Autodesk Inventor part; units mm, degrees
ref_plane "YZ Plane" through (0, 0, 0) normal (1, 0, 0) x (0, 1, 0)
ref_plane "XZ Plane" through (0, 0, 0) normal (0, 1, 0) x (-1, 0, 0)
ref_plane "XY Plane" through (0, 0, 0) normal (0, 0, 1) x (1, 0, 0)
sketch "スケッチ1" plane through (0, 0, 0) normal (0, 0, 1) x (1, 0, 0)
  line L0 (0, 0) -> (40, 0)
  line L1 (40, 0) -> (40, 318)
  line L2 (40, 318) -> (0, 318)
  line L3 (0, 318) -> (0, 0)
  line L4 (0, 218) -> (112.7627, 152.8964)
  line L5 (112.7627, 152.8964) -> (132.7627, 187.5375)
  line L6 (132.7627, 187.5375) -> (40, 241.094)
  point P0 (40, 218)
  point P1 (40, 194.906)
  point P2 (20, 318)
  point P3 (122.7627, 170.2169)
  point P4 (20, 258)
  dimension "d0" = 40
  dimension "d1" = 318
  dimension "d69" = 40
  dimension "d70" = 60
  dimension "d91" = 20
  dimension "d92" = 100
  dimension "d93" = 180
  dimension "d96" = 20
  dimension "d97" = 60
extrude "押し出し1" add sketch "スケッチ1" along normal blind 19.6 contours L3 L2 L1 L4 | L1 L6 L5 L4
sketch "スケッチ6" plane through (0, 0, 19.6) normal (0, 0, 1) x (1, 0, 0)
  circle A0 centre (20, 258) radius 4
  line L0 (40, 318) -> (0, 318)
  line L1 (40, 241.094) -> (40, 318)
  circle A1 centre (20, 20) radius 1.2295
  circle A2 centre (20, 10) radius 1.2295
  line L2 (0, 0) -> (40, 0)
  circle A3 centre (20, 298) radius 4
  point P0 (20, 318)
  point P1 (40, 190.8114)
  point P2 (30, 0)
  dimension "d42" = 8
  dimension "d44" = 20
  dimension "d45" = 2.459
  dimension "d46" = 2.459
  dimension "d47" = 10
  dimension "d48" = 10
  dimension "d49" = 20
  dimension "d50" = 20
  dimension "d53" = 8
  dimension "d54" = 20
  dimension "d55" = 40
  dimension "d56" = 20
extrude "押し出し4" cut sketch "スケッチ6" against normal through all
sketch "スケッチ8" plane through (0, 0, 0) normal (-1, 0, 0) x (0, 0, 1)
  line L0 (0, 318) -> (19.6, 318)
  line L1 (5, 318) -> (14.6, 318)
  line L2 (14.6, 318) -> (14.6, 278)
  line L3 (14.6, 278) -> (5, 278)
  line L4 (5, 278) -> (5, 318)
  line L5 (0, 318) -> (0, 0)
  dimension "d57" = 5
  dimension "d58" = 9.6
  dimension "d59" = 40
  dimension "d98" = 19.6
extrude "押し出し5" cut sketch "スケッチ8" against normal through all
fillet "フィレット1" radius 20 4 edges at (40, 318, 17.1) (40, 318, 2.5) (0, 318, 2.5) (0, 318, 17.1)
fillet "フィレット2" radius 40 2 edges at (0, 218, 9.8) (40, 241.094, 9.8)
sketch "スケッチ9" plane through (0, 0, 19.6) normal (0, 0, 1) x (1, 0, 0)
  line L0 (20, 206.453) -> (112.7627, 152.8964)
  line L1 (132.7627, 187.5375) -> (60, 229.547)
  line L2 (112.7627, 152.8964) -> (132.7627, 187.5375)
  line L3 (132.7627, 187.5375) -> (112.7627, 152.8964)
  line L4 (66.3813, 179.6747) -> (112.7627, 152.8964)
  line L5 (132.7627, 187.5375) -> (166.773, 167.9016)
  line L6 (115.1204, 126.9801) -> (133.5174, 158.8446)
  line L7 (141.7531, 173.1092) -> (128.7627, 180.6092)
  line L8 (112.7627, 152.8964) -> (20, 206.453)
  line L9 (132.7627, 187.5375) -> (60, 229.547)
  line L10 (115.1204, 126.9801) -> (125.7531, 145.3964)
  line L11 (133.5174, 158.8446) -> (145.7531, 180.0375)
  line L12 (116.7627, 159.8246) -> (129.7531, 152.3246)
  line L13 (66.3813, 179.6747) -> (129.7531, 152.3246)
  line L14 (66.3813, 179.6747) -> (86.3813, 214.3157)
  line L15 (86.3813, 214.3157) -> (141.7531, 173.1092)
  point P0 (0, 0)
  point P1 (254.4532, 80.329)
  point P2 (128.7627, 180.6092)
  point P3 (123.2579, 156.0746)
  point P4 (86.3813, 214.3157)
  point P5 (40, 194.906)
  point P6 (115.8875, 158.3088)
  point P7 (129.6379, 182.1251)
  dimension "d80" = 24
  dimension "d81" = 40
  dimension "d83" = 15
  dimension "d84" = 8
  dimension "d90" = 24
extrude "押し出し6" cut sketch "スケッチ9" against normal through all contours L13 L2 L0 | L1 L2 L15
sketch "スケッチ11" plane through (104.9897, 139.4332, 24) normal (0.8660254, -0.5, 0) x (0, 0, -1)
  line L0 (4.4, 21.7957) -> (4.4, 49.2964)
  line L1 (24, 21.7957) -> (24, 49.2964)
  line L2 (0, 24) -> (24, 24)
  line L3 (24, 24) -> (24, 0)
  line L4 (24, 0) -> (0, 0)
  line L5 (0, 0) -> (0, 24)
  line L6 (17, 17) -> (7, 17)
  line L7 (7, 17) -> (7, 7)
  line L8 (7, 7) -> (17, 7)
  line L9 (17, 7) -> (17, 17)
  line L10 (4.4, 35.546) -> (24, 35.546)
  circle A0 centre (14.2, 35.546) radius 5
  point P0 (24, -173.2475)
  point P1 (24, 24)
  point P2 (0, 15.546)
  point P3 (24, 15.546)
  dimension "d85" = 10
  dimension "d88" = 10
extrude "押し出し7" add sketch "スケッチ11" along normal blind 15 contours A0 L10 | L10 A0
fillet "フィレット4" radius 20 2 edges at (0, 278, 9.8) (40, 278, 9.8)
equation "\"d45\" = d46"
equation "\"d48\" = d47"
equation "\"d50\" = d49"
properties part number "legparts_06(seven)" material "ABS プラスチック"
The listing builds one solid part. Answer for the finished solid, in the listing's coordinates (mm). A direction names the side the tool comes from. Coordinates: 2 decimals unless noted, no trailing zeros. Loops run counter-clockwise (first coordinate to the right, second up) from the corner with the lowest first, then second, coordinate; pieces in that order, holes last. Notation, with made-up numbers: M 66.5,-32 L 80.5,-32 A15 ccw 80.5,-19 Z; hole C 54.25,36 d1. An arc over 180 degrees is marked long. Answer as CSV lines item,"result". Start each with the question number.
(1) The mould has two halves that part along Y. Classify faces 1 (the flat face through (0, 264, 3)), 2 (the flat face through (90.79, 169.14, 9.94)), 3 (the cylindrical face through (19.479, 261.966, 9.937)), 4 (the cylindrical face through (34.297, 311.986, 17.135)): pulls with the +Y half, pulls with the -Y half, needs draft (parallel to the pull), parting line crosses it, or undercut.
(2) The part is cut by section D-D (x = 14). Give the vertices of the cut face in (y, z), and give its area (3 significant figures).
(3) For faces 5 (the flat face through (40, 281, 17)), 6 (the flat face through (42.87, 193.25, 9.66)), 7 (the cylindrical face through (6.014, 272.297, 9.867)), 8 (the cylindrical face through (33.86, 272.72, 9.87)), 9 (the flat face through (50, 222, 0)), determine the directions among +Z, -Z, +X, -X, +Y, -Y from which every point of the face is accessible in a straight line to the end or side of a thin tool.
(4) The part is cut by section C-C (y = 248.5). Give the vertices of the cut face in (x, z), and give its area (3 significant figures).
(5) Given pin 1 (4 mm diameter, centred on y = 234, z = 3, fed in from +X); pin 2 (2.5 mm diameter, centred on y = 278, z = 2, fed in from +X); pin 3 (8 mm diameter, centred on y = 217.5, z = 13, fed in from -X); pin 4 (7 mm diameter, centred on x = 20, y = 258, fed in from -Z), each flat-ended and moving along its own axis, determine where each tip first touches the part or whether it passes through.
(6) Find the intervals of material crossed by L1, parallel to Y at x = 20, z = 15.9; L2, parallel to X at y = 298, z = 16.15; L3, parallel to Y at x = 20, z = 6.5, in increasing order. Write a range as [from, to].
(7) The part is cut by section B-B (x = 32). Give the vertices of the cut face in (y, z), and give its area (3 significant figures).
(8) The part is cut by section A-A (y = 291). Give the vertices of the cut face in (x, z), and give its area (3 significant figures).
Determined:
1,face 1,"needs draft"
1,face 2,"pulls with the -Y half"
1,face 3,"undercut"
1,face 4,"pulls with the +Y half"
2,outline,"M 210.7,0 L 317.08,0 L 317.08,5 L 277.08,5 L 277.08,14.6 L 317.08,14.6 L 317.08,19.6 L 210.7,19.6 Z"
2,area,"1,700 mm2"
3,face 5,"+Z, -Z, +X, +Y"
3,face 6,"+Z, -Z, -X, -Y"
3,face 7,"-X, +Y"
3,face 8,"+X, +Y"
3,face 9,"-Z, +X, -X, +Y, -Y"
4,outline,"M 0,0 L 43.2,0 L 43.2,19.6 L 0,19.6 Z"
4,area,"847 mm2"
5,pin 1,"x = 56.25"
5,pin 2,"x = 40"
5,pin 3,"x = 5.13"
5,pin 4,"through"
6,L1,"[206.45, 254], [262, 294], [302, 318]"
6,L2,"[0, 16], [24, 40]"
6,L3,"[206.45, 254], [262, 278]"
7,outline,"M 199.52,0 L 314,0 L 314,5 L 274.24,5 L 274.24,14.6 L 314,14.6 L 314,19.6 L 199.52,19.6 Z"
7,area,"1,860 mm2"
8,outline,"M 0,0 L 40,0 L 40,5 L 0,5 Z; M 0,14.6 L 40,14.6 L 40,19.6 L 0,19.6 Z"
8,area,"400 mm2"
